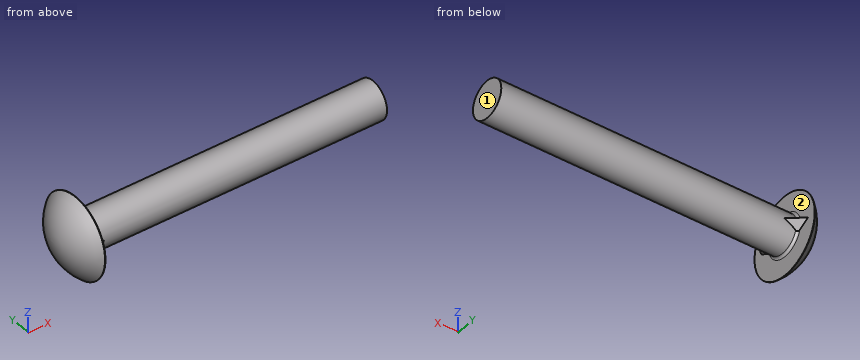
```python
from build123d import *

# Parameters (mm, degrees)
CIRPATTERN1_COUNT = 2


with BuildPart() as part:
    # ThreadSchematic: read off the stored shape, not the designer's step
    # ThreadSchematic outline → ThreadSchematic (revolve)
    with BuildSketch(Plane.YX):
        with BuildLine():
            Line((0, 108.204), (0, 0))
            ThreePointArc((0, 0), (7.486725405, 1.703037349), (13.500100004, 6.477000005))
            Line((13.500100004, 6.477000005), (13.5001, 6.604))
            Line((13.5001, 6.604), (7.1374, 6.604))
            ThreePointArc((7.1374, 6.604), (6.58062412, 6.83462412), (6.35, 7.3914))
            Line((6.35, 7.3914), (6.35, 108.204))
            Line((6.35, 108.204), (0, 108.204))
        make_face()
    revolve(axis=Axis((0, 0, 0), (1, 0, 0)))

    # Boss-Sweep2: sweep along a path in Sketch3
    with BuildLine(Plane.XY) as boss_sweep2_path:
        Line((6.604, 10.4521), (11.5062, 6.35))
    # Sketch4 → Boss-Sweep2 (sweep)
    with BuildSketch(Plane(origin=(6.604, 0, 0), x_dir=(0, 0, -1), z_dir=(1, 0, 0))):
        Polygon((0, 10.4521), (-2.5146, 5.830890742), (2.5146, 5.830890742), align=None)
    boss_sweep2 = sweep(path=boss_sweep2_path.line)

    # CirPattern1: Boss-Sweep2 ×2 about axis
    cirpattern1_axis = Axis((0, 0, 0), (1, 0, 0))
    for i in range(1, CIRPATTERN1_COUNT):
        add(boss_sweep2.rotate(cirpattern1_axis, i * 360 / CIRPATTERN1_COUNT))


solid = part.part
```
Design review of the part built by this model. Coordinates are the model's own, in mm. Face numbers are marked on the shaded views. A direction names the side the tool comes from. Round coordinates to 2 decimals unless told otherwise and drop trailing zeros. Order: outer loops, then holes, each group sorted by start corner. A loop starts at its lowest first (then second) coordinate and runs counter-clockwise, first axis right, second up. Notation, with made-up numbers: (35, 54.25) - (44, 54.25) arc R28 ccw to (44, 92.25) - close; hole circle Ø6 at (74, 27.25). An arc over 180 degrees is marked (long way). Return JSON: item names as keys, results as strings.
Q1. Wall thickness on L1, parallel to Y at x = 87.5, z = 0.5; L2, parallel to Z at x = 35, y = 4.25: over which ranges is each line inside the solid? List them lowest first. Write a range as [from, to].
Computed values:
{"L1": "y = [-6.33, 6.33]", "L2": "z = [-4.72, 4.72]"}
Q2. For pin 1 Ø2 at (x, z) = (27.5, -0.5) entering from -Y; pin 2 Ø4 at (x, z) = (78.5, -2.5) entering from +Y; pin 3 Ø1.5 at (x, y) = (51.5, 2.5) entering from +Z; pin 4 Ø13.5 at (y, z) = (6, -5.5) entering from +X, all flat-tipped, find the tip position at first contact; note any pin that passes through.
Computed values:
{"pin 1": "stops at y = -6.35", "pin 2": "stops at y = 6.33", "pin 3": "stops at z = 6.1", "pin 4": "stops at x = 108.2"}
Q3. Consider section B-B on x = 92. Write out the cut boundary in (y, z).
Computed values:
{"outline": "circle Ø12.7 at (0, 0)"}
Q4. Consider section C-C on z = 10.5. Write out the cut boundary in (x, y).
Computed values:
{"outline": "(6.48, -8.49) - (6.6, -8.49) - (6.6, 8.49) - (6.48, 8.49) arc R13.76 ccw to start"}
Q5. Consider section A-A on y = 0. Write out the cut boundary in (x, z), plus the area to 3 significant figures.
Computed values:
{"outline": "(6.48, -13.5) - (6.6, -13.5) - (6.6, -7.14) arc R0.79 cw to (7.39, -6.35) - (108.2, -6.35) - (108.2, 6.35) - (7.39, 6.35) arc R0.79 cw to (6.6, 7.14) - (6.6, 13.5) - (6.48, 13.5) arc R17.31 ccw to start", "area": "1,420 mm2"}
Q6. Consider section D-D on y = 9.25. Write out the cut boundary in (x, z), plus the area to 3 significant figures.
Computed values:
{"outline": "(6.48, -9.83) - (6.6, -9.83) - (6.6, -0.65) - (8.04, 0) - (6.6, 0.65) - (6.6, 9.83) - (6.48, 9.83) arc R14.63 ccw to start", "area": "54.7 mm2"}
Q7. Machinability: for the marked faces 1 and 2, which of the approach directions +Z, -Z, +X, -X, +Y, -Y give a long, thin tool a straight path to every point of the face, cutting with its end or side? Answer none if there is none.
Computed values:
{"face 1": "+Z, -Z, +X, +Y, -Y", "face 2": "+X"}
